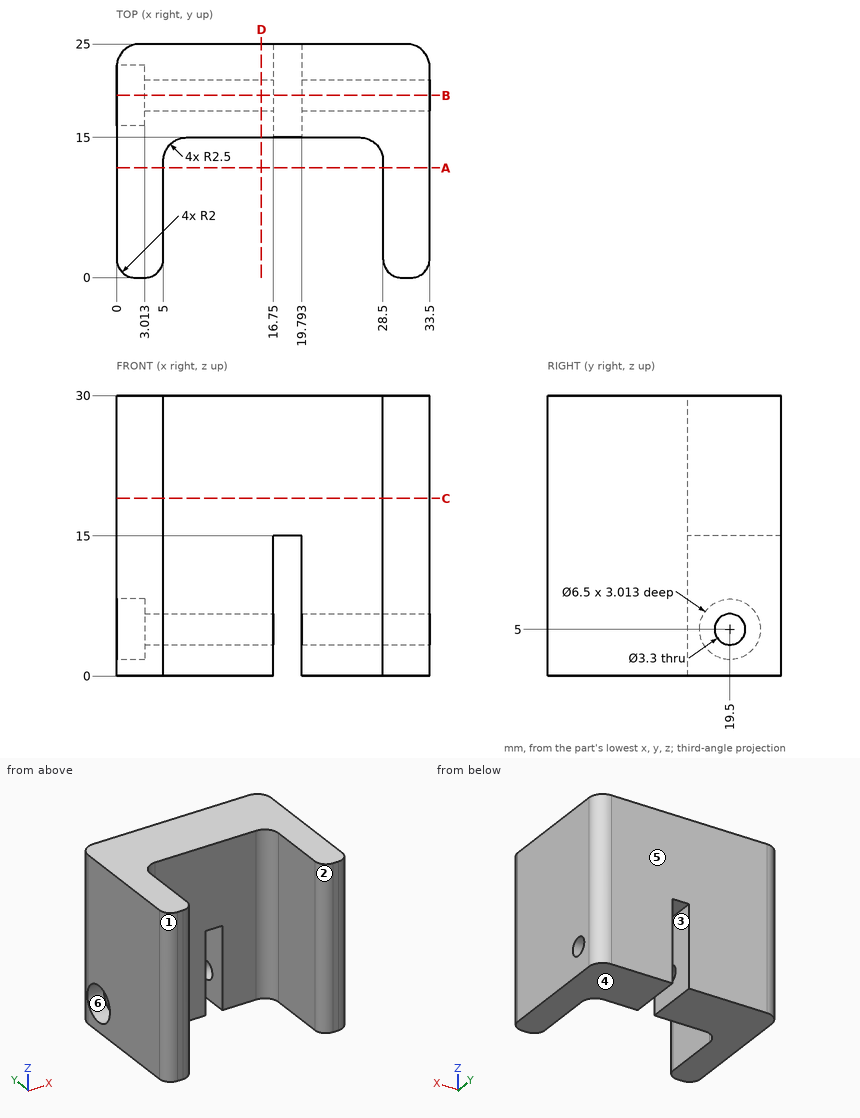
Answer from the drawing. Dimensions are ordinates in mm from the lowest x, y and z of the part. A direction names the side the tool comes from. Round coordinates to 2 decimals unless told otherwise and drop trailing zeros. Write each loop counter-clockwise with the first axis right and the second up, starting at its lowest first coordinate (ties: lowest second). Pieces come first, ordered by that corner, then holes. Notation, with made-up numbers: (-27, 7.5) -> (21, 7.5) arc R24 ccw to (21, 32.5) -> close; hole circle Ø8 at (-23.75, 17). An arc over 180 degrees is marked (long way). Answer in a Markdown table with one row per item. Add a question column.
1) Determine the mould class of the marked faces 4, 5 and 6 for opening direction Z: pulls with the +Z half, pulls with the -Z half, needs draft (parallel to the pull), parting line crosses it, or undercut.
2) Find section C-C, the plane z = 19. Determine the outline of the cut face in (x, y).
3) Find section D-D, the plane x = 15.5. Determine the outline of the cut face in (y, z).
4) Given P1, Ø2.5, axis at y = 19.5, z = 5, coming from the +X side; P2, Ø7, axis at y = 18.5, z = 3.5, coming from the -X side; P3, Ø5.5, axis at x = 15.5, z = 15, coming from the -Y side; P4, Ø5, axis at y = 19.5, z = 5, coming from the -X side, each flat-ended and moving along its own axis, determine where each tip first touches the part or whether it passes through.
5) Find section A-A, the plane y = 11.75. Determine the outline of the cut face in (x, z).
6) Consider line 1 (X direction, y = 4.25, z = 28.5); line 2 (Z direction, x = 1.85, y = 19.5); line 3 (X direction, y = 20.75, z = 3). Determine where each line is inside the solid, lowest interval first.
7) Which of the six approach directions +Z, -Z, +X, -X, +Y, -Y give full straight-line access (tool end or side, diameter ignored) to the marked faces 1, 2 and 3?
8) Find section B-B, the plane y = 19.5. Determine the outline of the cut face in (x, z), and give its area (3 significant figures).
Findings below:
| question | item | result |
|---|---|---|
| 1 | face 4 | pulls with the -Z half |
| 1 | face 5 | needs draft |
| 1 | face 6 | undercut |
| 2 | outline | (0, 2) arc R2 ccw to (2, 0) -> (3, 0) arc R2 ccw to (5, 2) -> (5, 12.5) arc R2.5 cw to (7.5, 15) -> (26, 15) arc R2.5 cw to (28.5, 12.5) -> (28.5, 2) arc R2 ccw to (30.5, 0) -> (31.5, 0) arc R2 ccw to (33.5, 2) -> (33.5, 22.5) arc R2.5 ccw to (31, 25) -> (2.5, 25) arc R2.5 ccw to (0, 22.5) -> close |
| 3 | outline | (15, 0) -> (25, 0) -> (25, 30) -> (15, 30) -> close; hole circle Ø3.3 at (19.5, 5) |
| 4 | P1 | through |
| 4 | P2 | x = 0 |
| 4 | P3 | y = 15 |
| 4 | P4 | x = 3.01 |
| 5 | outline | (0, 0) -> (5, 0) -> (5, 30) -> (0, 30) -> close; (28.5, 0) -> (33.5, 0) -> (33.5, 30) -> (28.5, 30) -> close |
| 6 | line 1 | 0 to 5, 28.5 to 33.5 |
| 6 | line 2 | 0 to 1.75, 8.25 to 30 |
| 6 | line 3 | 3.01 to 16.75, 19.79 to 33.5 |
| 7 | face 1 | +Z, -Z, -X, -Y |
| 7 | face 2 | +Z, -Z, -Y |
| 7 | face 3 | -Z, +Y, -Y |
| 8 | outline | (0, 0) -> (16.75, 0) -> (16.75, 3.35) -> (3.01, 3.35) -> (3.01, 1.75) -> (0, 1.75) -> close; (0, 8.25) -> (3.01, 8.25) -> (3.01, 6.65) -> (16.75, 6.65) -> (16.75, 15) -> (19.79, 15) -> (19.79, 6.65) -> (33.5, 6.65) -> (33.5, 30) -> (0, 30) -> close; (19.79, 0) -> (33.5, 0) -> (33.5, 3.35) -> (19.79, 3.35) -> close |
| 8 | area | 849 mm² |
